```python
from build123d import *

# Parameters (mm, degrees)
BOSS_EXTRUDE1_DEPTH = 4


with BuildPart() as part:
    # Sketch1 → Boss-Extrude1 (new body)
    with BuildSketch(Plane.XY):
        with BuildLine():
            Line((7.7, 0), (15, 0))
            ThreePointArc((15, 0), (19, -4), (23, 0))
            Line((23, 0), (65, 0))
            ThreePointArc((65, 0), (69, -4), (73, 0))
            Line((73, 0), (80.3, 0))
            Line((80.3, 0), (80.3, 20))
            Line((80.3, 20), (84, 20))
            Line((84, 20), (84, 0))
            Line((84, 0), (88, 0))
            Line((88, 0), (88, 40))
            Line((88, 40), (73, 40))
            ThreePointArc((73, 40), (69, 36), (65, 40))
            Line((65, 40), (23, 40))
            ThreePointArc((23, 40), (19, 36), (15, 40))
            Line((15, 40), (0, 40))
            Line((0, 40), (0, 0))
            Line((0, 0), (4, 0))
            Line((4, 0), (4, 20))
            Line((4, 20), (7.7, 20))
            Line((7.7, 20), (7.7, 0))
        make_face()
    extrude(amount=BOSS_EXTRUDE1_DEPTH)


solid = part.part
```
The listing builds one solid part. Answer for the finished solid, in the listing's coordinates (mm). A direction names the side the tool comes from. Round coordinates to 2 decimals unless told otherwise and drop trailing zeros. Loops run counter-clockwise (first coordinate to the right, second up) from the corner with the lowest first, then second, coordinate; pieces in that order, holes last. Notation, with made-up numbers: (3, -6) - (17, -6) arc R16 cw to (17, 24) - close; hole circle Ø6 at (-24.75, 57). An arc over 180 degrees is marked (long way). Return JSON: item names as keys, results as strings. Group by question number.
1. The part is cut by section B-B on z = 2.85. Determine the outline of the cut face in (x, y), then the cut area to 3 significant figures.
2. Consider probe 1 along X at (y, z) = (16.5, 3.8); probe 2 along Y at (x, z) = (61, 0.3); probe 3 along Y at (x, z) = (67, 0.6). Determine where each line is inside the solid, lowest interval first.
3. Each of these flat-tipped pins is pushed along its axis until it touches: P1, Ø2, axis at x = 1, z = 2.5, coming from the -Y side; P2, Ø1.1, axis at x = 81, z = 1, coming from the -Y side. Where does it stop, or does it pass through?
4. Which of the six approach directions +Z, -Z, +X, -X, +Y, -Y give full straight-line access (tool end or side, diameter ignored) to faces 5 (the flat face through (44, 40, 2)), 6 (the flat face through (11, 0, 2)), 7 (the flat face through (80.3, 10, 2)), 8 (the flat face through (77, 0, 2)), 9 (the flat face through (43, 23, 4))?
5. The mould has two halves that part along X. Classify faces 1 (the flat face through (88, 20, 2)), 2 (the flat face through (43, 23, 0)), 3 (the cylindrical face through (19, -4, 2)), 4 (the cylindrical face through (19, 36, 2)): pulls with the +X half, pulls with the -X half, needs draft (parallel to the pull), parting line crosses it, or undercut.
6. The part is cut by section C-C on x = 69. Determine the outline of the cut face in (y, z), then the cut area to 3 significant figures.
7. The part is cut by section A-A on y = 18. Determine the outline of the cut face in (x, z).
Resolved:
{
 "1": {"outline": "(0, 0) - (4, 0) - (4, 20) - (7.7, 20) - (7.7, 0) - (15, 0) arc R4 ccw to (23, 0) - (65, 0) arc R4 ccw to (73, 0) - (80.3, 0) - (80.3, 20) - (84, 20) - (84, 0) - (88, 0) - (88, 40) - (73, 40) arc R4 cw to (65, 40) - (23, 40) arc R4 cw to (15, 40) - (0, 40) - close", "area": "3,370 mm²"},
 "2": {"probe 1": "x = 0 to 4, 7.7 to 80.3, 84 to 88", "probe 2": "y = 0 to 40", "probe 3": "y = -3.46 to 36.54"},
 "3": {"P1": "stops at y = 0", "P2": "stops at y = 20"},
 "4": {"face 5": "+Z, -Z, +X, -X, +Y", "face 6": "+Z, -Z, -X, -Y", "face 7": "+Z, -Z, -Y", "face 8": "+Z, -Z, +X, -Y", "face 9": "+Z, +X, -X, +Y, -Y"},
 "5": {"face 1": "pulls with the +X half", "face 2": "needs draft", "face 3": "undercut", "face 4": "undercut"},
 "6": {"outline": "(-4, 0) - (36, 0) - (36, 4) - (-4, 4) - close", "area": "160 mm²"},
 "7": {"outline": "(0, 0) - (4, 0) - (4, 4) - (0, 4) - close; (7.7, 0) - (80.3, 0) - (80.3, 4) - (7.7, 4) - close; (84, 0) - (88, 0) - (88, 4) - (84, 4) - close"}
}
